from build123d import *

# Parameters (mm, degrees)
SKETCH_R     = 22.5
PAD_DEPTH    = 25
SKETCH001_R  = 6.164928
POCKET_DEPTH = 96.547437


with BuildPart() as part:
    # Sketch → Pad (new body, symmetric)
    with BuildSketch(Plane.XZ):
        with BuildLine():
            ThreePointArc((-28.726667, 24.104535), (0, -37.5), (28.726667, 24.104535))
            ThreePointArc((40, 56.546437), (25.155668, 43.525085), (28.726667, 24.104535))
            Line((40, 56.546437), (40, 96.546437))
            Line((30, 96.546437), (40, 96.546437))
            Line((6.164928, 76.546437), (30, 96.546437))
            Line((-6.164928, 76.546437), (6.164928, 76.546437))
            Line((-30, 96.546437), (-6.164928, 76.546437))
            Line((-40, 96.546437), (-30, 96.546437))
            Line((-40, 56.546437), (-40, 96.546437))
            ThreePointArc((-28.726667, 24.104535), (-25.155668, 43.525085), (-40, 56.546437))
        make_face()
        Circle(SKETCH_R, mode=Mode.SUBTRACT)
    extrude(amount=PAD_DEPTH, both=True)

    # Sketch001 → Pocket (cut, through all)
    with BuildSketch(Plane.XY):
        Circle(SKETCH001_R)
    extrude(amount=POCKET_DEPTH, mode=Mode.SUBTRACT)


solid = part.part
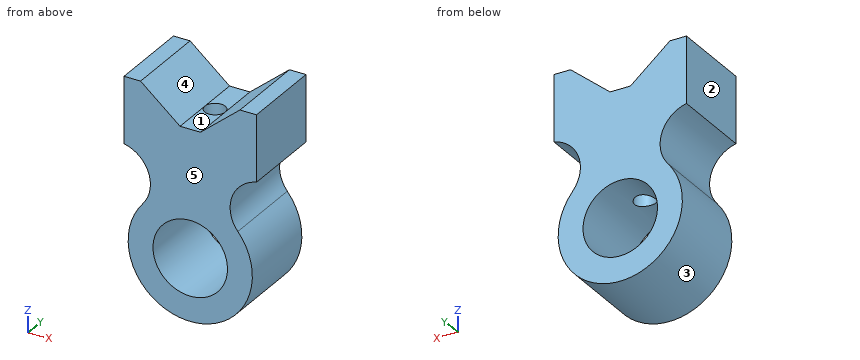
Verification items for the finished model (mm, model axes). Face numbers are marked on the shaded views. A direction names the side the tool comes from. Give positions to 0.01 mm unless a question says otherwise; leave off trailing zeros. Loops run counter-clockwise (first coordinate to the right, second up) from the corner with the lowest first, then second, coordinate; pieces in that order, holes last.
1) Sectioned sample at B-B, the plane z = 0. Enter the section's corners in (x, y).
2) Depth check by flat-ended pin: pin 1 Ø12 at (y, z) = (-19.5, -17) entering from -X; pin 2 Ø10 at (x, y) = (-2, -14.5) entering from +Z; pin 3 Ø10 at (x, y) = (-2.5, 18.5) entering from +Z. Enter the tip coordinate at first touch or a pass-through.
3) Sectioned sample at C-C, the plane y = 11. Enter the section's corners in (x, z), then the cut area to 3 significant figures.
4) Sectioned sample at D-D, the plane x = 17.5. Enter the section's corners in (y, z), then the cut area to 3 significant figures.
5) Thickness scan on line 1 along X through (y, z) = (0, 64); line 2 along Y through (x, z) = (0, 55); line 3 along X through (y, z) = (0, 38). Record the ranges inside material, lowest first.
6) Draft check along Z on the marked faces 3, 4 and 5. Enter one of: pulls with the +Z half, pulls with the -Z half, needs draft (parallel to the pull), parting line crosses it, or undercut.
7) Set-up check for the marked faces 1 and 2: record each of +Z, -Z, +X, -X, +Y, -Y from which the full face is reachable in a straight line by a thin tool's end or side.
8) Sectioned sample at A-A, the plane x = 0. Enter the section's corners in (y, z).
Answers:
1. outline: (-37.5, -25) - (-22.5, -25) - (-22.5, 25) - (-37.5, 25) - close; (22.5, -25) - (37.5, -25) - (37.5, 25) - (22.5, 25) - close
2. pin 1: stops at x = -35.85
2. pin 2: stops at z = 77.25
2. pin 3: stops at z = 77.67
3. outline: (-40, 56.55) arc R20 cw to (-28.73, 24.1) arc R37.5 ccw (long way) to (28.73, 24.1) arc R20 cw to (40, 56.55) - (40, 96.55) - (30, 96.55) - (6.16, 76.55) - (-6.16, 76.55) - (-30, 96.55) - (-40, 96.55) - close; hole circle Ø45 at (0, 0)
3. area: 6,530 mm2
4. outline: (-25, -33.17) - (25, -33.17) - (25, -14.14) - (-25, -14.14) - close; (-25, 14.14) - (25, 14.14) - (25, 86.06) - (-25, 86.06) - close
4. area: 4,550 mm2
5. line 1: x = -40 to -6.16, 6.16 to 40
5. line 2: y = -25 to -6.16, 6.16 to 25
5. line 3: x = -24.07 to -6.16, 6.16 to 24.07
6. face 3: undercut
6. face 4: pulls with the +Z half
6. face 5: needs draft
7. face 1: +Z, +Y, -Y
7. face 2: +Z, -Z, -X, +Y, -Y
8. outline: (-25, -37.5) - (25, -37.5) - (25, -22.5) - (-25, -22.5) - close; (-25, 22.5) - (-6.16, 22.5) - (-6.16, 76.55) - (-25, 76.55) - close; (6.16, 22.5) - (25, 22.5) - (25, 76.55) - (6.16, 76.55) - close
